Check sheet for the drawn part. Datum: minimum x, y, z corner. Units: mm. Give positions to 0.01 mm unless a question says otherwise; leave off trailing zeros. Order: outer loops, then holes, each group sorted by start corner. A loop starts at its lowest first (then second) coordinate and runs counter-clockwise, first axis right, second up. Notation, with made-up numbers: (7, 53.5) -> (45, 53.5) arc R31 cw to (45, 83.5) -> close; hole circle Ø11 at (14.25, 11). An arc over 180 degrees is marked (long way). Return JSON: item names as keys, results as strings. Group by question number.
(1) Cross-section at B-B on x = 14.5. Enter the section's corners in (y, z) (1 decimal).
(2) Depth check by flat-ended pin: pin 1 Ø1.5 at (x, y) = (19, 2) entering from +Z. Enter the tip coordinate at first touch or a pass-through.
(3) Thickness scan on line 1 along X through (y, z) = (2.4, 31) (1 decimal); line 2 along X through (y, z) = (0.3, 25); line 3 along Z through (x, y) = (8, 1.75). Record the ranges inside material, lowest first.
(4) Cross-section at C-C on z = 3. Enter the section's corners in (x, y) (1 decimal), then the cut area to 3 significant figures.
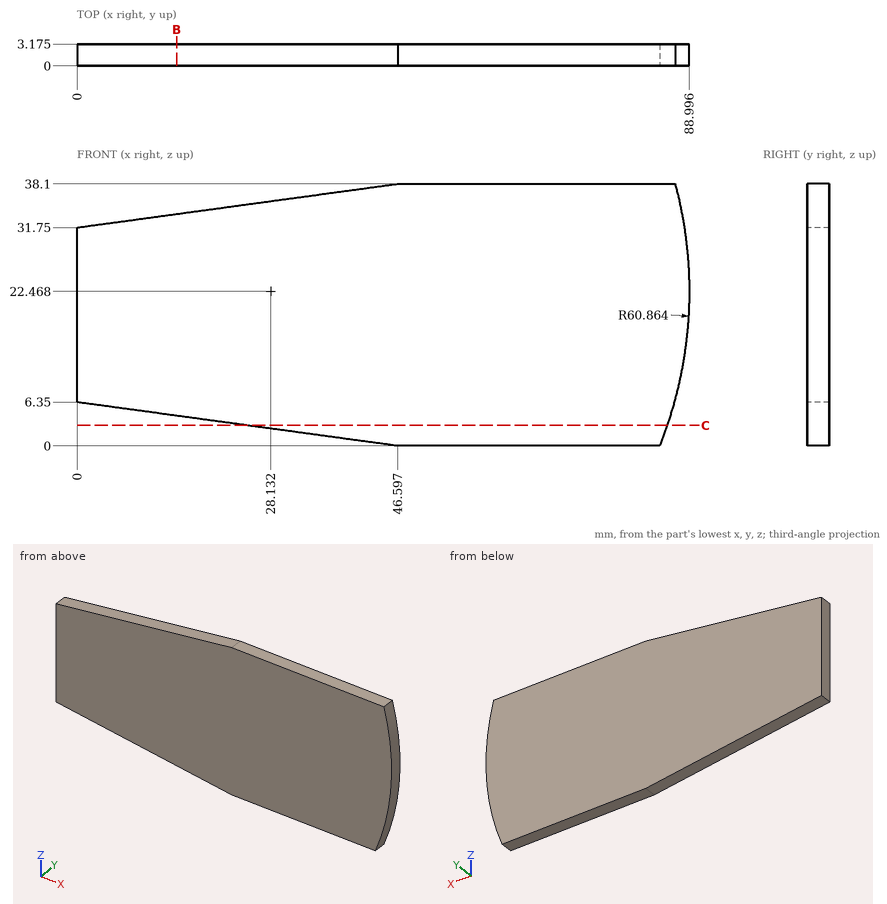
Verdict:
{
 "1": {"outline": "(0, 4.4) -> (3.2, 4.4) -> (3.2, 33.7) -> (0, 33.7) -> close"},
 "2": {"pin 1": "z = 34.44"},
 "3": {"line 1": "0 to 88.4", "line 2": "0 to 88.94", "line 3": "5.26 to 32.84"},
 "4": {"outline": "(24.6, 0) -> (85.8, 0) -> (85.8, 3.2) -> (24.6, 3.2) -> close", "area": "194 mm²"}
}
